Here's how the part is built. I have some questions about the finished solid (model axes, mm). Face numbers are marked on the shaded views. Round coordinates to 2 decimals unless told otherwise and drop trailing zeros. Order: outer loops, then holes, each group sorted by start corner. A loop starts at its lowest first (then second) coordinate and runs counter-clockwise, first axis right, second up. Notation, with made-up numbers: M 11,62 L 44,62 A18 ccw 44,96 Z; hole C -24,-22.75 d5. An arc over 180 degrees is marked long. Answer as CSV lines item,"result". Start each with the question number.
```python
from build123d import *

# Parameters (mm, degrees)
SKETCH1_W           = 50
SKETCH1_H           = 170.451051634
BOSS_EXTRUDE1_DEPTH = 282
CUT_EXTRUDE1_DEPTH  = 8
CUT_EXTRUDE2_DEPTH  = 5
FILLET3_R           = 5
SKETCH5_R           = 3.175
CUT_EXTRUDE3_DEPTH  = 7.7
CUT_EXTRUDE4_START  = -7.7
SKETCH6_R           = 3.175
CUT_EXTRUDE4_DEPTH  = 7.7
FILLET4_R           = 5


with BuildPart() as part:
    # Sketch1 → Boss-Extrude1 (new body)
    with BuildSketch(Plane.XY):
        with Locations((-197.021929301, 35.225525817)):
            Rectangle(SKETCH1_W, SKETCH1_H)
        Polygon((0, -50), (0, 0), (-172.021929301, 120.451051634), (-172.021929301, -50), align=None)
    extrude(amount=BOSS_EXTRUDE1_DEPTH)

    # Sketch3 → Cut-Extrude1 (cut)
    with BuildSketch(Plane(origin=(0, 0, 0), x_dir=(0.819152044288989, -0.5735764363510502, 0), z_dir=(0.5735764363510502, 0.819152044288989, 0))):
        Polygon((-37.234042553, -232), (-172.765957447, -50), (-172.765957447, -232), align=None)
        Polygon((-37.234042553, -50), (-172.765957447, -50), (-37.234042553, -232), align=None)
    extrude(amount=-CUT_EXTRUDE1_DEPTH, mode=Mode.SUBTRACT)

    # Sketch4 → Cut-Extrude2 (cut)
    with BuildSketch(Plane(origin=(0, 120.451051634, 0), x_dir=(1, 0, 0), z_dir=(0, 1, 0))):
        Polygon((-202.021929301, -112.8), (-192.021929301, -169.2), (-192.021929301, -16), (-202.021929301, -16), align=None)
        Polygon((-192.021929301, -266), (-192.021929301, -169.2), (-202.021929301, -112.8), (-202.021929301, -266), align=None)
    extrude(amount=-CUT_EXTRUDE2_DEPTH, mode=Mode.SUBTRACT)

    # Fillet3
    # the kernel refuses this fillet: 5 mm, written as the material it adds along each edge
    with BuildSketch(Plane(origin=(-197.021929301, 120.451051634, 261), x_dir=(0, 0, 1), z_dir=(0, -1, 0))) as fillet3_piece_1_section:
        Polygon((0, 0), (FILLET3_R * 1.02, 0), (FILLET3_R * 1.02, FILLET3_R * 1.02), (0, FILLET3_R * 1.02), align=None)
    fillet3_piece_1 = extrude(amount=FILLET3_R * 1.02, mode=Mode.PRIVATE)
    fillet3_piece_1 = fillet3_piece_1 - Plane(origin=(-197.021929301, 120.451051634, 261), x_dir=(0.7071067811865475, 0, -0.7071067811865475), z_dir=(0, -1, 0)) * Sphere(FILLET3_R, mode=Mode.PRIVATE)
    with BuildSketch(Plane(origin=(-197.021929301, 120.451051634, 21), x_dir=(0, -1, 0), z_dir=(0, 0, -1))) as fillet3_piece_2_section:
        Polygon((0, 0), (FILLET3_R * 1.02, 0), (FILLET3_R * 1.02, FILLET3_R * 1.02), (0, FILLET3_R * 1.02), align=None)
    fillet3_piece_2 = extrude(amount=FILLET3_R * 1.02, mode=Mode.PRIVATE)
    fillet3_piece_2 = fillet3_piece_2 - Plane(origin=(-197.021929301, 120.451051634, 21), x_dir=(0.7071067811865474, 0.7071067811865478, 0), z_dir=(0, 0, -1)) * Sphere(FILLET3_R, mode=Mode.PRIVATE)
    with BuildSketch(Plane(origin=(-197.021929301, 120.451051634, 261), x_dir=(0, 0, 1), z_dir=(1, 0, 0))) as fillet3_piece_3_section:
        Polygon((0, 0), (FILLET3_R * 1.02, 0), (FILLET3_R * 1.02, FILLET3_R * 1.02), (0, FILLET3_R * 1.02), align=None)
    fillet3_piece_3 = extrude(amount=FILLET3_R * 1.02, mode=Mode.PRIVATE)
    fillet3_piece_3 = fillet3_piece_3 - Plane(origin=(-197.021929301, 120.451051634, 261), x_dir=(0, 0.7071067811865475, -0.7071067811865475), z_dir=(1, 0, 0)) * Sphere(FILLET3_R, mode=Mode.PRIVATE)
    with BuildSketch(Plane(origin=(-197.021929301, 120.451051634, 21), x_dir=(1, 0, 0), z_dir=(0, 0, -1))) as fillet3_piece_4_section:
        Polygon((0, 0), (FILLET3_R * 1.02, 0), (FILLET3_R * 1.02, FILLET3_R * 1.02), (0, FILLET3_R * 1.02), align=None)
    fillet3_piece_4 = extrude(amount=FILLET3_R * 1.02, mode=Mode.PRIVATE)
    fillet3_piece_4 = fillet3_piece_4 - Plane(origin=(-197.021929301, 120.451051634, 21), x_dir=(-0.7071067811865478, 0.7071067811865474, 0), z_dir=(0, 0, -1)) * Sphere(FILLET3_R, mode=Mode.PRIVATE)
    with BuildSketch(Plane(origin=(-192.021929301, 115.451051634, 261), x_dir=(0, 1, 0), z_dir=(0, 0, -1))) as fillet3_piece_5:
        with BuildLine():
            CenterArc((FILLET3_R, -FILLET3_R), FILLET3_R, 90, 90)
            Line((0, -FILLET3_R), (0, 0))
            Line((0, 0), (FILLET3_R, 0))
        make_face()
    fillet3_piece_5_solid = extrude(amount=240, mode=Mode.PRIVATE)
    with BuildSketch(Plane(origin=(-202.021929301, 115.451051634, 261), x_dir=(0, 1, 0), z_dir=(0, 0, -1))) as fillet3_piece_6:
        with BuildLine():
            CenterArc((FILLET3_R, FILLET3_R), FILLET3_R, 180, 90)
            Line((0, FILLET3_R), (0, 0))
            Line((0, 0), (FILLET3_R, 0))
        make_face()
    fillet3_piece_6_solid = extrude(amount=240, mode=Mode.PRIVATE)
    add([fillet3_piece_1, fillet3_piece_2, fillet3_piece_3, fillet3_piece_4, fillet3_piece_5_solid, fillet3_piece_6_solid])

    # Sketch5 → Cut-Extrude3 (cut)
    with BuildSketch(Plane.XY.offset(282)):
        with Locations((-52.5, -32.5)):
            Circle(SKETCH5_R)
        with Locations((-169.521929301, -32.5)):
            Circle(SKETCH5_R)
    extrude(amount=-CUT_EXTRUDE3_DEPTH, mode=Mode.SUBTRACT)

    # Sketch6 → Cut-Extrude4 (cut)
    with BuildSketch(Plane(origin=(0, 0, 0), x_dir=(-1, 0, 0), z_dir=(0, 0, -1)).offset(CUT_EXTRUDE4_START)):
        with Locations(Location((169.521929301, -32.5, 0), (0, 0, 180))):
            Circle(SKETCH6_R)
        with Locations(Location((52.5, -32.5, 0), (0, 0, 180))):
            Circle(SKETCH6_R)
    extrude(amount=CUT_EXTRUDE4_DEPTH, mode=Mode.SUBTRACT)

    # Fillet4
    fillet4_edges = [part.edges().sort_by_distance(p)[0] for p in [
        (-222.021929301, 35.225525817, 282),
        (-172.021929301, 120.451051634, 141),
        (0, 0, 141),
        (-222.021929301, 120.451051634, 141),
        (0, -25, 282),
        (-86.01096465, 60.225525817, 282),
        (-197.021929301, 120.451051634, 282),
        (-86.01096465, 60.225525817, 0),
        (0, -25, 0),
        (-222.021929301, 35.225525817, 0),
        (-197.021929301, 120.451051634, 0),
    ]]
    fillet(fillet4_edges, radius=FILLET4_R)


solid = part.part
```
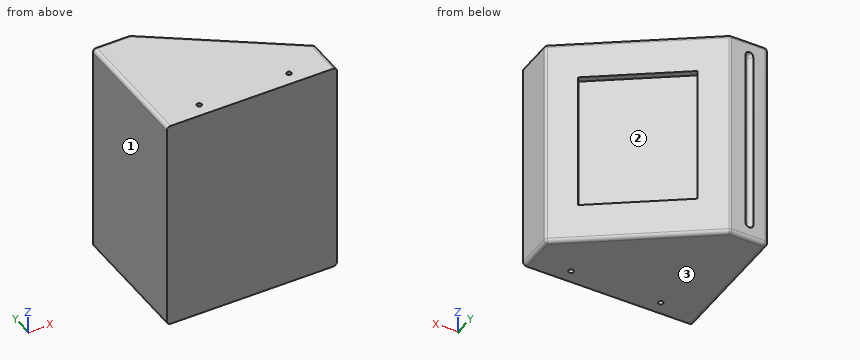
Item 1: For P1, Ø3, axis at x = -62.5, z = 236, coming from the +Y side; P2, Ø3, axis at x = -169.5, y = -32, coming from the +Z side; P3, Ø4, axis at x = -52.5, y = -32.5, coming from the -Z side, each with a flat end and sliding along its axis, tell me the tip position at first contact or that it passes through.
Item 2: If I drill on line 1 along X through (y, z) = (-32, 277); line 2 along X through (y, z) = (-32.5, 3.5) (3 decimals); line 3 along Y through (x, z) = (-52.5, 278) (3 decimals), over which ranges is the centre line in solid material (lowest first)?
Item 3: We'd pull the mould along Z, two halves only. Please class the marked faces 1, 2 and 3: pulls with the +Z half, pulls with the -Z half, needs draft (parallel to the pull), parting line crosses it, or undercut.
Item 4: If we section it at A-A on z = 228.5: Please give me the cut outline in (x, y), and give its area (3 significant figures).
Geometry says:
1,P1,"y = 44.81"
1,P2,"z = 274.3"
1,P3,"z = 7.7"
2,line 1,"-222.02 to -172.66, -166.39 to -55.64, -49.36 to 0"
2,line 2,"-221.792 to -172.697, -166.347 to -55.675, -49.325 to -0.23"
2,line 3,"-50 to -35.675, -29.325 to 36.638"
3,face 1,"needs draft"
3,face 2,"undercut"
3,face 3,"pulls with the -Z half"
4,outline,"M -222.02,-50 L 0,-50 L 0,-2.6 A5 ccw -2.13,1.49 L -30.5,21.36 L -35.09,14.8 L -146.11,92.54 L -141.52,99.09 L -170.73,119.55 A5 ccw -173.6,120.45 L -192.02,120.45 A5 cw -202.02,120.45 L -217.02,120.45 A5 ccw -222.02,115.45 Z"
4,area,"26,400 mm²"
